Design review of the part built by this model. Coordinates are the model's own, in mm. Round coordinates to 2 decimals unless told otherwise and drop trailing zeros. Order: outer loops, then holes, each group sorted by start corner. A loop starts at its lowest first (then second) coordinate and runs counter-clockwise, first axis right, second up. Notation, with made-up numbers: (21.25, -30.75) - (53.25, -30.75) arc R16 cw to (53.25, -26.75) - close; hole circle Ø6 at (68, 31.5). An arc over 180 degrees is marked (long way). Use CSV: the item, a comma, the result in double quotes. Start each with the question number.
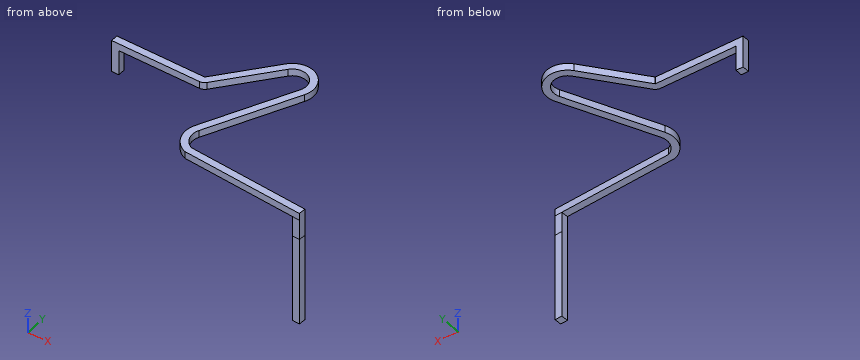
from build123d import *

# Parameters (mm, degrees)
Y_KSEKLIK_EKSTR_ZYON1_DEPTH = 2.8
IZIM2_W                     = 2.8
IZIM2_H                     = 2.8
Y_KSEKLIK_EKSTR_ZYON3_DEPTH = 45
Y_KSEKLIK_EKSTR_ZYON4_DEPTH = 8
IZIM4_W                     = 2.8
IZIM4_H                     = 2.803743846
KES_EKSTR_ZYON1_DEPTH       = 35
Y_KSEKLIK_EKSTR_ZYON5_DEPTH = 35


with BuildPart() as part:
    # Çizim1 → Yükseklik-Ekstrüzyon1 (new body)
    with BuildSketch(Plane.XY):
        with BuildLine():
            Line((0, 0), (34.587072671, 0))
            ThreePointArc((34.587072671, 0), (35.865324826, 0.285949258), (36.899900144, 1.089285714))
            Line((36.899900144, 1.089285714), (53.833333333, 21.586389745))
            ThreePointArc((53.833333333, 21.586389745), (61.045741484, 22.711143216), (63.022721024, 15.684376278))
            Line((63.022721024, 15.684376278), (46.447554388, -18.510124025))
            ThreePointArc((46.447554388, -18.510124025), (46.197115168, -25.807507473), (51.434005635, -30.895680351))
            Line((51.434005635, -30.895680351), (99.127590258, -34.315623722))
            Line((99.127590258, -34.315623722), (99.327854452, -31.522794645))
            Line((99.327854452, -31.522794645), (52.068910631, -28.134017876))
            ThreePointArc((52.068910631, -28.134017876), (48.729396862, -24.592999144), (48.967149147, -19.731452093))
            Line((48.967149147, -19.731452093), (65.542315784, 14.46304821))
            ThreePointArc((65.542315784, 14.46304821), (62.558873931, 25.067078316), (51.674694359, 23.369723078))
            Line((51.674694359, 23.369723078), (34.741261169, 2.872619048))
            ThreePointArc((34.741261169, 2.872619048), (34.672289482, 2.819063284), (34.587072671, 2.8))
            Line((34.587072671, 2.8), (0, 2.8))
            Line((0, 2.8), (0, 0))
        make_face()
    extrude(amount=Y_KSEKLIK_EKSTR_ZYON1_DEPTH)

    # Çizim2 → Yükseklik-Ekstrüzyon3 (add)
    with BuildSketch(Plane(origin=(0, 0, 0), x_dir=(-1, 0, 0), z_dir=(0, 0, -1))):
        with Locations((-1.4, 1.4)):
            Rectangle(IZIM2_W, IZIM2_H)
    extrude(amount=Y_KSEKLIK_EKSTR_ZYON3_DEPTH)

    # Çizim3 → Yükseklik-Ekstrüzyon4 (add)
    with BuildSketch(Plane(origin=(0, 0, 0), x_dir=(-1, 0, 0), z_dir=(0, 0, -1))):
        Polygon((-99.327854452, -31.522794645), (-99.127590258, -34.315623722), (-96.334761181, -34.115359528), (-96.535025375, -31.322530451), align=None)
    extrude(amount=Y_KSEKLIK_EKSTR_ZYON4_DEPTH)

    # Çizim4 → Kes-Ekstrüzyon1 (cut)
    with BuildSketch(Plane(origin=(0, 0, -45), x_dir=(-1, 0, 0), z_dir=(0, 0, -1))):
        with Locations((-1.4, 1.398128077)):
            Rectangle(IZIM4_W, IZIM4_H)
    extrude(amount=-KES_EKSTR_ZYON1_DEPTH, mode=Mode.SUBTRACT)

    # Çizim5 → Yükseklik-Ekstrüzyon5 (add)
    with BuildSketch(Plane(origin=(0, 0, -8), x_dir=(-1, 0, 0), z_dir=(0, 0, -1))):
        Polygon((-96.535025375, -31.322530451), (-96.334761181, -34.115359528), (-99.127284523, -34.315601799), (-99.327548717, -31.522772722), align=None)
    extrude(amount=Y_KSEKLIK_EKSTR_ZYON5_DEPTH)


solid = part.part
Q1. Take a section at D-D (x = 24). State the section outline as (y, z) points, plus the area to 3 significant figures.
Q2. Take a section at A-A (z = -2.5). State the section outline as (x, y) points.
Q3. Clearance check with flat-ended pins moving along their axes: pin 1 (14 mm diameter, centred on x = 13.5, z = -3, fed in from +Y); pin 2 (2 mm diameter, centred on y = 17, z = -2.5, fed in from -X); pin 3 (1.4 mm diameter, centred on x = 1.5, y = 1, fed in from -Z); pin 4 (12 mm diameter, centred on x = 60, y = -2, fed in from -Z). State where each tip first meets the part, or that it passes through.
Q4. Take a section at C-C (x = 55). State the section outline as (y, z) points, plus the area to 3 significant figures.
Q5. Take a section at B-B (y = 9.5). State the section outline as (x, z) points, plus the area to 3 significant figures.
Findings below:
1,outline,"(0, 0) - (2.8, 0) - (2.8, 2.8) - (0, 2.8) - close"
1,area,"7.84 mm^2"
2,outline,"(0, 0) - (2.8, 0) - (2.8, 2.8) - (0, 2.8) - close; (96.33, -34.12) - (99.13, -34.32) - (99.33, -31.52) - (96.54, -31.32) - close"
3,pin 1,"stops at y = 2.8"
3,pin 2,"passes through"
3,pin 3,"stops at z = -10"
3,pin 4,"stops at z = 0"
4,outline,"(-31.15, 0) - (-28.34, 0) - (-28.34, 2.8) - (-31.15, 2.8) - close; (-7.29, 0) - (-0.87, 0) - (-0.87, 2.8) - (-7.29, 2.8) - close; (22.64, 0) - (25.79, 0) - (25.79, 2.8) - (22.64, 2.8) - close"
4,area,"34.7 mm^2"
5,outline,"(40.22, 0) - (43.85, 0) - (43.85, 2.8) - (40.22, 2.8) - close; (60.02, 0) - (63.14, 0) - (63.14, 2.8) - (60.02, 2.8) - close"
5,area,"18.9 mm^2"
